Can you work these out from the model? Positions are in its coordinate system, mm. Coordinates: 2 decimals unless noted, no trailing zeros.
```python
from build123d import *

# Parameters (mm, degrees)
SKETCH1_R           = 1.65
BOSS_EXTRUDE1_DEPTH = 5
SKETCH4_W           = 28.7
SKETCH4_H           = 5.5
BOSS_EXTRUDE3_DEPTH = 5
SKETCH5_R           = 1.65
CUT_EXTRUDE2_DEPTH  = 6
SKETCH6_R           = 1.65
CUT_EXTRUDE3_DEPTH  = 6
FILLET1_R           = 5


with BuildPart() as part:
    # Sketch1 → Boss-Extrude1 (new body)
    with BuildSketch(Plane(origin=(0, 0, 0), x_dir=(1, 0, 0), z_dir=(0, 1, 0))):
        Polygon((0, 0), (227, 0), (259, 0), (259, 22), (227, 22), (0, 22), align=None)
        with Locations((230.5, 19)):
            Circle(SKETCH1_R, mode=Mode.SUBTRACT)
        with Locations((255.5, 19)):
            Circle(SKETCH1_R, mode=Mode.SUBTRACT)
        with Locations((30.5, 19)):
            Circle(SKETCH1_R, mode=Mode.SUBTRACT)
        with Locations((55.5, 19)):
            Circle(SKETCH1_R, mode=Mode.SUBTRACT)
        with Locations((8.5, 11)):
            Circle(SKETCH1_R, mode=Mode.SUBTRACT)
        with Locations((18.5, 18.5)):
            Circle(SKETCH1_R, mode=Mode.SUBTRACT)
        with Locations((18.5, 3.5)):
            Circle(SKETCH1_R, mode=Mode.SUBTRACT)
    extrude(amount=BOSS_EXTRUDE1_DEPTH)

    # Sketch4 → Boss-Extrude3 (add)
    with BuildSketch(Plane(origin=(0, 5, 0), x_dir=(1, 0, 0), z_dir=(0, 1, 0))):
        with Locations((43.05, -2.75)):
            Rectangle(SKETCH4_W, SKETCH4_H)
        with Locations((100.45, -2.75)):
            Rectangle(SKETCH4_W, SKETCH4_H)
        with Locations((157.85, -2.75)):
            Rectangle(SKETCH4_W, SKETCH4_H)
        with Locations((215.25, -2.75)):
            Rectangle(SKETCH4_W, SKETCH4_H)
    extrude(amount=-BOSS_EXTRUDE3_DEPTH)

    # Sketch5 → Cut-Extrude2 (cut, through all)
    with BuildSketch(Plane(origin=(0, 5, 0), x_dir=(1, 0, 0), z_dir=(0, 1, 0))):
        with Locations((28.7, 0)):
            Circle(SKETCH5_R)
        with Locations((57.4, 0)):
            Circle(SKETCH5_R)
        with Locations((86.1, 0)):
            Circle(SKETCH5_R)
        with Locations((114.8, 0)):
            Circle(SKETCH5_R)
        with Locations((143.5, 0)):
            Circle(SKETCH5_R)
        with Locations((172.2, 0)):
            Circle(SKETCH5_R)
        with Locations((200.9, 0)):
            Circle(SKETCH5_R)
        with Locations((229.6, 0)):
            Circle(SKETCH5_R)
    extrude(amount=-CUT_EXTRUDE2_DEPTH, mode=Mode.SUBTRACT)

    # Sketch6 → Cut-Extrude3 (cut, through all)
    with BuildSketch(Plane(origin=(0, 5, 0), x_dir=(1, 0, 0), z_dir=(0, 1, 0))):
        with Locations((75.8, 11)):
            Circle(SKETCH6_R)
        with Locations((92.6, 11)):
            Circle(SKETCH6_R)
        with Locations((109.4, 11)):
            Circle(SKETCH6_R)
        with Locations((126.2, 11)):
            Circle(SKETCH6_R)
        with Locations((143, 11)):
            Circle(SKETCH6_R)
        with Locations((159.8, 11)):
            Circle(SKETCH6_R)
        with Locations((176.6, 11)):
            Circle(SKETCH6_R)
        with Locations((193.4, 11)):
            Circle(SKETCH6_R)
        with Locations((210.2, 11)):
            Circle(SKETCH6_R)
    extrude(amount=-CUT_EXTRUDE3_DEPTH, mode=Mode.SUBTRACT)

    # Fillet1
    fillet1_edges = [part.edges().sort_by_distance(p)[0] for p in [
        (259, 2.5, -22),
    ]]
    fillet(fillet1_edges, radius=FILLET1_R)


solid = part.part
```
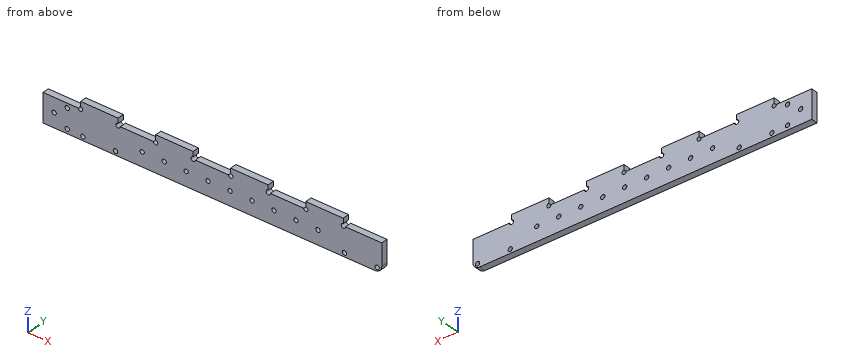
1. Please list where these lines run through material, in increasing order: probe 1 along X at (y, z) = (4.05, 2.25); probe 2 along Z at (x, y) = (55.5, 3.65); probe 3 along X at (y, z) = (3.35, -3.5).
Completed:
probe 1: x = 28.7 to 57.4, 86.1 to 114.8, 143.5 to 172.2, 200.9 to 229.6
probe 2: z = -22 to -20.65, -17.35 to 5.5
probe 3: x = 0 to 16.85, 20.15 to 259
2. Imagine slicing it at A-A on y = 2.75. Give the number of separate pieces and of enclosed holes in the cut face, then the cut area to 3 significant figures.
Completed:
separate pieces: 1
enclosed holes: 16
area: 6,140 mm2
3. I'm going to push flat-ended pins straight in: pin 1 (1.2 mm diameter, centred on y = 2, z = 4, fed in from +X); pin 2 (3 mm diameter, centred on y = 3.5, z = 4, fed in from -X); pin 3 (2.5 mm diameter, centred on x = 19, y = 1.5, fed in from +Z); pin 4 (1 mm diameter, centred on y = 3, z = -11.5, fed in from -X). Where does each tip first touch, or does it pass through?
Completed:
pin 1: stops at x = 229.6
pin 2: stops at x = 28.7
pin 3: stops at z = 0
pin 4: stops at x = 0
